Part print with two shaded views. Sizes in mm from the minimum x, y, z corner. Give positions to 0.01 mm unless a question says otherwise; leave off trailing zeros. Write each loop counter-clockwise with the first axis right and the second up, starting at its lowest first coordinate (ties: lowest second). Pieces come first, ordered by that corner, then holes. Notation, with made-up numbers: (75.5, 86.25) -> (105.5, 86.25) arc R33 cw to (105.5, 121.25) -> close; hole circle Ø6 at (61.5, 88). An arc over 180 degrees is marked (long way). Use one line per item in the form item = value. Start each with the question number.
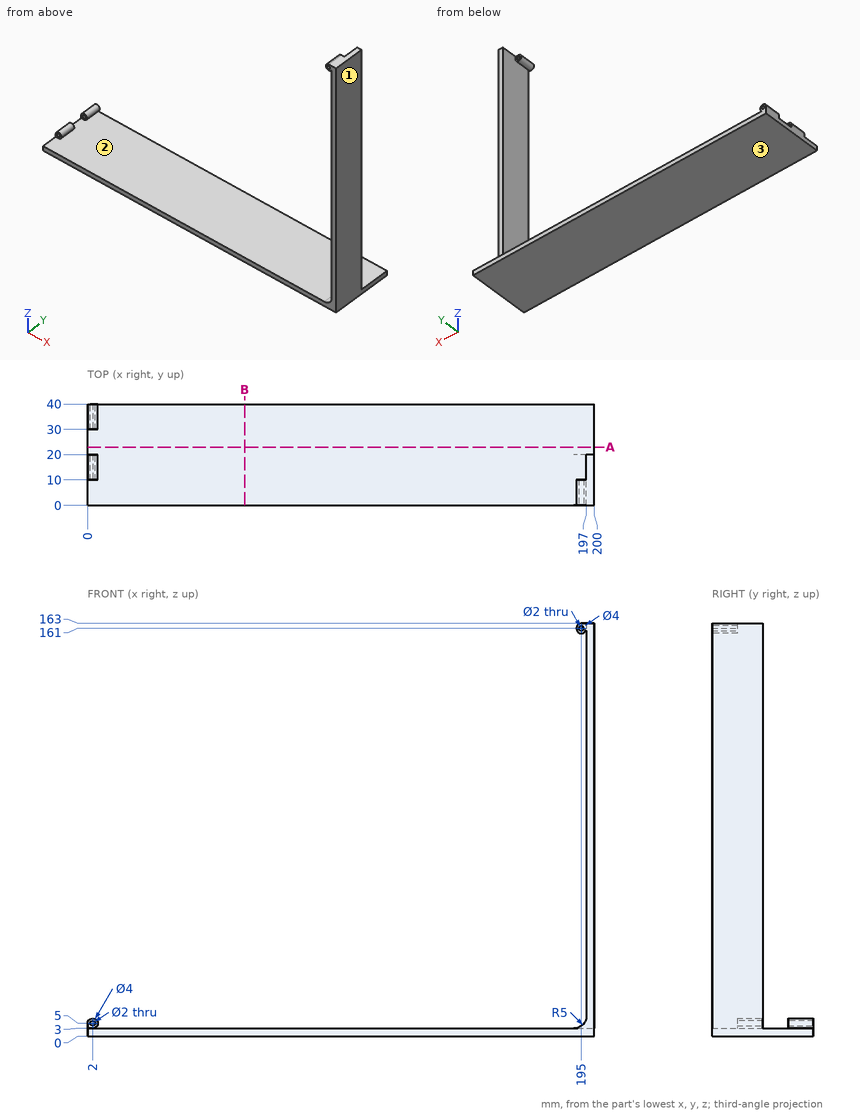
1) Wall check: line 1 along X through (y, z) = (12.75, 5); line 2 along X through (y, z) = (32.5, 5); line 3 along Z through (x, y) = (21.5, 28.5). Give the ranges that are in metal, low to high. Write a range as from..to.
2) Cut at B-B (x = 62). Give the cut face in (y, z), and give its area (3 significant figures).
3) Two-plate mould, pull along X, no slides. Class the marked faces 1, 2 and 3: released by +X, released by -X, zero draft, split by the parting line, or undercut.
4) Pin check, flat tips, straight feed: pin 1 (3 mm diameter, centred on x = 1, z = 5.5, fed in from -Y); pin 2 (8 mm diameter, centred on x = 139.5, y = 33.5, fed in from +Z); pin 3 (1.2 mm diameter, centred on x = 195, z = 160.5, fed in from +Y). Stop position of each tip, or through.
5) Cut at A-A (y = 23). Give the cut face in (x, z), and give its area (3 significant figures).
Final values:
q1.line_1 = 0..1, 3..4, 196..200
q1.line_2 = 0..1, 3..4
q1.line_3 = 0..3
q2.outline = (0, 0) -> (40, 0) -> (40, 3) -> (0, 3) -> close
q2.area = 120 mm^2
q3.face_1 = released by +X
q3.face_2 = undercut
q3.face_3 = zero draft
q4.pin_1 = 10
q4.pin_2 = 3
q4.pin_3 = 10
q5.outline = (0, 0) -> (200, 0) -> (200, 3) -> (0, 3) -> close
q5.area = 600 mm^2
